For this review, take the finished solid that the model builds, in its own axes (mm). Face numbers are marked on the shaded views. A direction names the side the tool comes from. Round coordinates to 2 decimals unless told otherwise and drop trailing zeros. Loops run counter-clockwise (first coordinate to the right, second up) from the corner with the lowest first, then second, coordinate; pieces in that order, holes last.
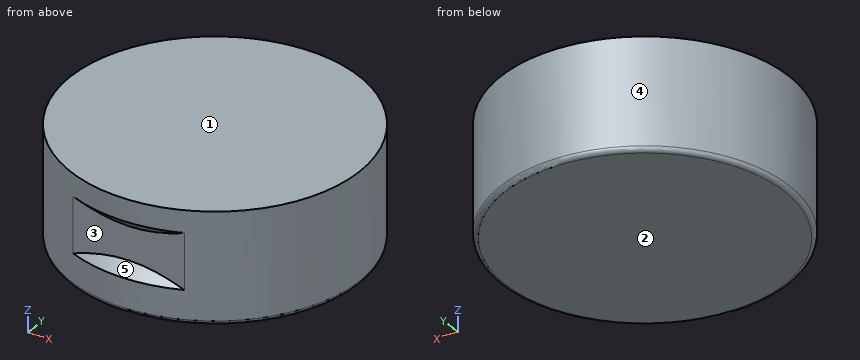
```python
from build123d import *

# Parameters (mm, degrees)
F0_R     = 65
F1_DEPTH = 50
F2_R     = 2
F4_W     = 50
F4_H     = 15
F5_DEPTH = 25
F6_SIZE  = 4.99999


# Not quite as in the source:
# - a fillet or chamfer is up to 0.001 mm smaller than in the source, because OpenCascade refuses the exact size


with BuildPart() as f1:
    # F0 (on Top) → F1 (new body)
    with BuildSketch(Plane.XY):
        Circle(F0_R)
    extrude(amount=F1_DEPTH)

    # F2
    f2_edges = [f1.edges().sort_by_distance(p)[0] for p in [
        (-65, 0, 0),
    ]]
    fillet(f2_edges, radius=F2_R)

    # F4 (on offset) → F5 (cut)
    with BuildSketch(Plane.XZ.offset(60)):
        with Locations((0, 27.5)):
            Rectangle(F4_W, F4_H)
    extrude(amount=F5_DEPTH, mode=Mode.SUBTRACT)

    # F6 (size 5 in the source; OpenCascade refuses exactly that, so slightly less here)
    f6_edges = [f1.edges().sort_by_distance(p)[0] for p in [
        (0, -65, 20),
        (0, -65, 35),
    ]]
    chamfer(f6_edges, length=F6_SIZE)


solid = f1.part
```
(1) For the marked faces 4 and 5, list the 3-axis set-ups (+Z, -Z, +X, -X, +Y, -Y) from which the entire face can be reached by the end or side of a thin tool; tool diameter is ignored.
(2) For L1, parallel to X at y = -16, z = 10.5; L2, parallel to X at y = -0.5, z = 19.5; L3, parallel to Y at x = -41.5, z = 11, list the stretches that pass through material, from the lowest coordinate up.
(3) Add section A-A (z = 7). Give the boundary of the cut face in (x, y), plus the area to 3 significant figures.
(4) Insertion check: pin 1 Ø5 at (x, z) = (39.5, 30.5) entering from -Y; pin 2 Ø5 at (x, z) = (-12, 26.5) entering from +Y; pin 3 Ø5 at (y, z) = (-12, 42) entering from +X. Each pin has a flat end and moves straight along its axis. Give the tip position at first contact, or say it passes through.
(5) Add section B-B (z = 17). Give the boundary of the cut face in (x, y), plus the area to 3 significant figures.
(6) The part is to be moulded in two halves that separate along Z. For the marked faces 1, 2 and 3, say which applies: pulls with the +Z half, pulls with the -Z half, needs draft (parallel to the pull), parting line crosses it, or undercut.
Outcome:
1. face 4: +Z, -Z
1. face 5: -Y
2. L1: x = -63 to 63
2. L2: x = -65 to 65
2. L3: y = -50.03 to 50.03
3. outline: circle Ø130 at (0, 0)
3. area: 13,300 mm2
4. pin 1: stops at y = -53.44
4. pin 2: stops at y = 64.3
4. pin 3: stops at x = 64.3
5. outline: (-25, -60) - (-19.21, -60) arc R63 ccw to (19.21, -60) - (25, -60) arc R65 ccw (long way) to start
5. area: 13,200 mm2
6. face 1: pulls with the +Z half
6. face 2: pulls with the -Z half
6. face 3: undercut
